Read the model definition and answer for the solid it produces. Units are mm, in the model's axes. Coordinates: 2 decimals unless noted, no trailing zeros. Order: outer loops, then holes, each group sorted by start corner. A loop starts at its lowest first (then second) coordinate and runs counter-clockwise, first axis right, second up. Notation, with made-up numbers: M 50,39.25 L 77,39.25 A31 ccw 77,77.25 Z; hole C -6,83 d7. An arc over 180 degrees is marked long. One line per question, with ' | ' between items. Start each with the question number.
1) Find section A-A, the plane y = 23. Write down the section's boundary in (x, z).
2) Given P1, Ø1.6, axis at x = -4.5, y = -29, coming from the +Z side; P2, Ø0.6, axis at x = 0.5, y = -29, coming from the +Z side; P3, Ø1, axis at y = 7.5, z = 39.5, coming from the -X side, each flat-ended and moving along its own axis, determine where each tip first touches the part or whether it passes through.
3) Consider probe 1 along X at (y, z) = (-21.5, 66); probe 2 along X at (y, z) = (-3, 62); probe 3 along X at (y, z) = (-8.5, 24). Determine where each line is inside the solid, lowest interval first.
4) Find section B-B, the plane z = 25. Write down the section's boundary in (x, y), plus the area to 3 significant figures.
5) Find section C-C, the plane x = 22. Write down the section's boundary in (y, z).
from build123d import *

# Parameters (mm, degrees)
F1_DEPTH      = 30
F1_DEPTH_BACK = 30
F3_DEPTH      = 30
F3_DEPTH_BACK = 30
F5_DEPTH      = 2


with BuildPart() as f1:
    # F0 (on Front) → F1 (new body, two sides)
    with BuildSketch(Plane.XZ) as f1_sk:
        Polygon((-25, 70), (-25, 0), (0, 0), (25, 0), (25, 70), (0, 102.580634), align=None)
    extrude(amount=F1_DEPTH)
    extrude(f1_sk.sketch, amount=-F1_DEPTH_BACK)

    # F2 (on Front) → F3 (join, two sides)
    with BuildSketch(Plane.XZ) as f3_sk:
        Polygon((-33.481879, 62.23156), (-31.895172, 61.014037), (0, 102.580634), (31.895172, 61.014037), (33.481879, 62.23156), (0, 105.865994), align=None)
    extrude(amount=F3_DEPTH)
    extrude(f3_sk.sketch, amount=-F3_DEPTH_BACK)

    # F4 (on face) → F5 (cut)
    with BuildSketch(Plane.XZ.offset(30)):
        with BuildLine():
            Line((-7, 72), (-3, 72))
            ThreePointArc((-3, 72), (-2.902414, 72.758942), (-2.616005, 73.468509))
            Line((-2.616005, 73.468509), (-6.104012, 75.42652))
            ThreePointArc((-6.104012, 75.42652), (-6.7723, 73.770864), (-7, 72))
        make_face()
        with BuildLine():
            Line((-5.553473, 76.26133), (-2.38006, 73.826284))
            ThreePointArc((-2.38006, 73.826284), (-1.422173, 74.641481), (-0.214286, 74.992337))
            Line((-0.214286, 74.992337), (-0.5, 78.98212))
            ThreePointArc((-0.5, 78.98212), (-3.318405, 78.163456), (-5.553473, 76.26133))
        make_face()
        with BuildLine():
            ThreePointArc((5.553473, 76.26133), (3.318405, 78.163456), (0.5, 78.98212))
            Line((0.5, 78.98212), (0.214286, 74.992337))
            ThreePointArc((0.214286, 74.992337), (1.422173, 74.641481), (2.38006, 73.826284))
            Line((2.38006, 73.826284), (5.553473, 76.26133))
        make_face()
        with BuildLine():
            ThreePointArc((7, 72), (6.7723, 73.770864), (6.104012, 75.42652))
            Line((6.104012, 75.42652), (2.616005, 73.468509))
            ThreePointArc((2.616005, 73.468509), (2.902414, 72.758942), (3, 72))
            Line((3, 72), (7, 72))
        make_face()
        with BuildLine():
            ThreePointArc((-1.744003, 72.979006), (-1.934943, 72.505961), (-2, 72))
            Line((-2, 72), (0, 72))
            Line((0, 72), (2, 72))
            ThreePointArc((2, 72), (1.934943, 72.505961), (1.744003, 72.979006))
            ThreePointArc((1.744003, 72.979006), (1.66962, 73.101077), (1.586707, 73.217523))
            ThreePointArc((1.586707, 73.217523), (0.948116, 73.760987), (0.142857, 73.994891))
            ThreePointArc((0.142857, 73.994891), (0, 74), (-0.142857, 73.994891))
            ThreePointArc((-0.142857, 73.994891), (-0.948116, 73.760987), (-1.586707, 73.217523))
            ThreePointArc((-1.586707, 73.217523), (-1.66962, 73.101077), (-1.744003, 72.979006))
        make_face()
    extrude(amount=-F5_DEPTH, mode=Mode.SUBTRACT)


solid = f1.part
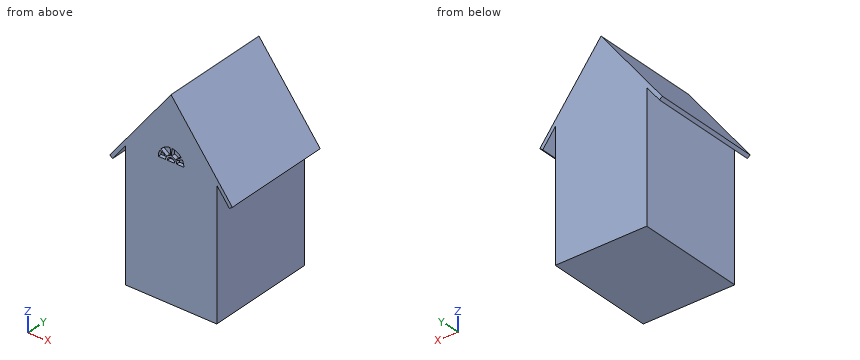
Report:
1) outline: M -33.48,62.23 L -31.9,61.01 L -25,70 L -25,0 L 25,0 L 25,70 L 31.9,61.01 L 33.48,62.23 L 0,105.87 Z
2) P1: stops at z = 101.04 | P2: stops at z = 105.61 | P3: stops at x = -25
3) probe 1: x = -30.59 to -28.07, -25 to 25, 28.07 to 30.59 | probe 2: x = -33.18 to -31.14, -25 to 25, 31.14 to 33.18 | probe 3: x = -25 to 25
4) outline: M -25,-30 L 25,-30 L 25,30 L -25,30 Z | area: 3,000 mm^2
5) outline: M -30,0 L 30,0 L 30,77.2 L -30,77.2 Z
